Job drawing, mm, ordinate dimensions from the low corner. One solid piece. A direction names the side the tool comes from. Round coordinates to 2 decimals unless told otherwise and drop trailing zeros. Loops run counter-clockwise (first coordinate to the right, second up) from the corner with the lowest first, then second, coordinate; pieces in that order, holes last.
1) Band-saw the part on C-C, the plane y = 5.5. State how many separate pieces and enclosed holes the cut face has, then the cut area to 3 significant figures.
2) Band-saw the part on D-D, the plane z = 23.8. Write the cut outline in (x, y) (1 decimal).
3) Band-saw the part on A-A, the plane z = 12.8. Write the cut outline in (x, y).
4) 3-axis set-ups, long thin cutter, end or side, ignore diameter. For the marked faces 5 and 6: which of +Z, -Z, +X, -X, +Y, -Y reach the whole face in a straight line?
5) Band-saw the part on B-B, the plane x = 23.8. Write the cut outline in (y, z) (1 decimal).
6) Mould opens along Z. For the marked faces 1, 2, 3 and 4 say: +Z half, -Z half, draft (parallel to the pull), parting line (faces both ways), or undercut.
7) Drop flat-ended pins along their axis: P1, Ø3, axis at x = 12.8, z = 1.8, coming from the +Y side; P2, Ø9, axis at x = 12.8, z = 12.8, coming from the -Y side; P3, Ø1, axis at y = 3.5, z = 6, coming from the -X side. Give the stop position or say it passes through.
8) Probe line 1 (Z direction, x = 12.8, y = 5); line 2 (X direction, y = 2.25, z = 21) (1 decimal); line 3 (Y direction, x = 16.5, z = 5.25). List the from-to ranges inside material, lowest first.
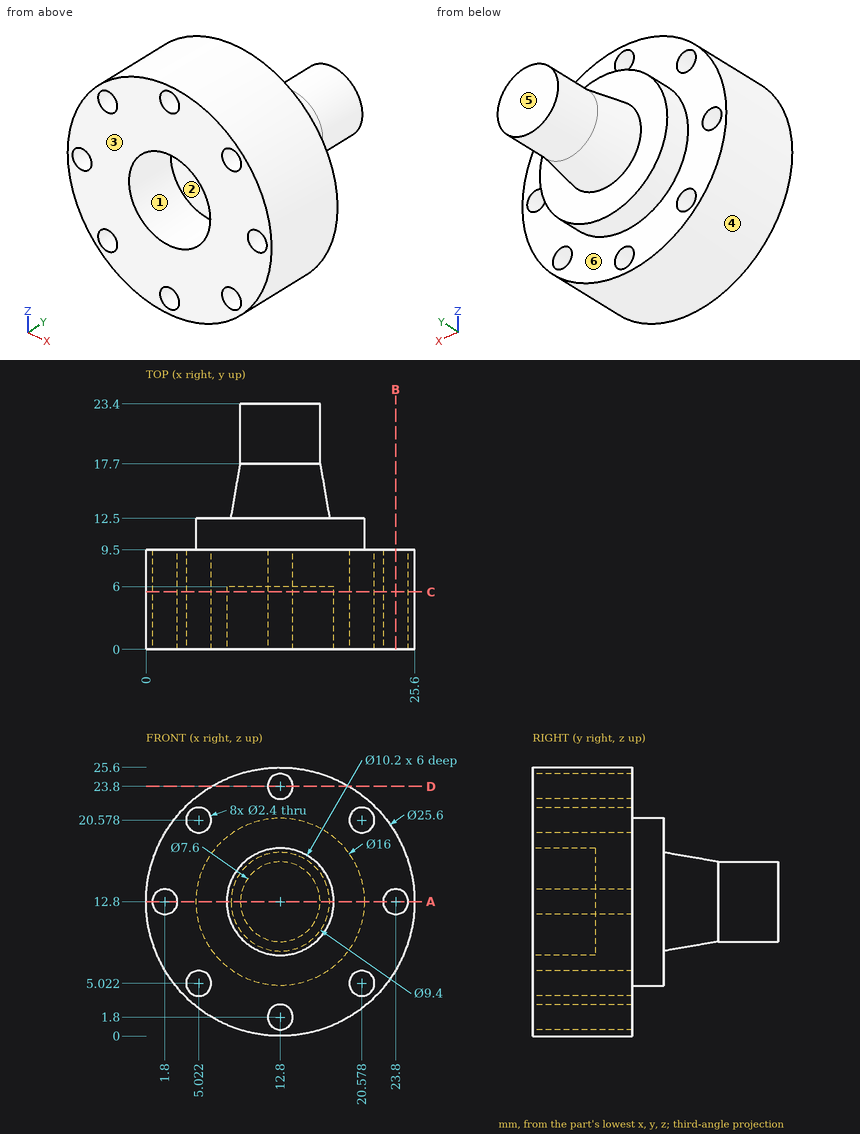
Reported:
1. separate pieces: 1
1. enclosed holes: 9
1. area: 397 mm2
2. outline: (6.3, 0) - (11.6, 0) - (11.6, 9.5) - (6.3, 9.5) - close; (14, 0) - (19.3, 0) - (19.3, 9.5) - (14, 9.5) - close
3. outline: (0, 0) - (0.6, 0) - (0.6, 9.5) - (0, 9.5) - close; (3, 0) - (7.7, 0) - (7.7, 6) - (17.9, 6) - (17.9, 0) - (22.6, 0) - (22.6, 9.5) - (20.8, 9.5) - (20.8, 12.5) - (17.5, 12.5) - (16.6, 17.7) - (16.6, 23.4) - (9, 23.4) - (9, 17.7) - (8.1, 12.5) - (4.8, 12.5) - (4.8, 9.5) - (3, 9.5) - close; (25, 0) - (25.6, 0) - (25.6, 9.5) - (25, 9.5) - close
4. face 5: +Z, -Z, +X, -X, +Y
4. face 6: +Y
5. outline: (0, 6.3) - (9.5, 6.3) - (9.5, 11.6) - (0, 11.6) - close; (0, 14) - (9.5, 14) - (9.5, 19.3) - (0, 19.3) - close
6. face 1: undercut
6. face 2: undercut
6. face 3: draft
6. face 4: parting line
7. P1: stops at y = 9.5
7. P2: stops at y = 6
7. P3: stops at x = 1.66
8. line 1: z = 0 to 0.6, 3 to 7.7, 17.9 to 22.6, 25 to 25.6
8. line 2: x = 3 to 3.9, 6.1 to 19.5, 21.7 to 22.6
8. line 3: y = 0 to 9.5
